Autodesk Inventor part; units mm, degrees
ref_plane "Work Plane2" through (12.9398, -24.5988, -20.5) normal (0, 0, 1) x (0.7071087, 0.7071049, 0)
ref_plane "YZ Plane" through (0, 0, 0) normal (1, 0, 0) x (0, 1, 0)
ref_plane "XZ Plane" through (0, 0, 0) normal (0, 1, 0) x (-1, 0, 0)
ref_plane "Work Plane1" through (69.3531, 0, -24) normal (0, 0, -1) x (-0.9792327, -0.2027397, 0)
sketch "Sketch1" plane through (69.3531, 0, -24) normal (0, 0, -1) x (-0.9792327, -0.2027397, 0)
  circle A0 centre (8.0687, 11.3576) radius 25.9979
  circle A1 centre (8.0703, 11.3562) radius 3.8103
  circle A2 centre (8.0703, 11.3562) radius 5
  point P0 (67.9128, 14.0606)
  dimension "d0" = 10
extrude "Extrusion1" add sketch "Sketch1" along normal blind 4 contours A0
sketch "Sketch2" plane through (59.1493, 9.4859, -28) normal (0, 0, -1) x (-1, 0, 0)
  line L0 (59.1493, -50.593) -> (59.1493, 54.0449)
  line L1 (-54.0467, -9.4859) -> (50.5907, -9.4859)
  line L2 (-15.9479, -15.1669) -> (4.4725, 20.2023)
  line L3 (4.4725, 20.2023) -> (19.4213, 5.2535)
  line L4 (19.4213, 5.2535) -> (-15.9479, -15.1669)
  line L5 (-39.0985, 39.0967) -> (35.6425, -35.6447)
  line L6 (-0.781, 0) -> (9.2905, 10.0715)
  line L7 (-0.781, 0) -> (13.4622, 0) construction
  line L8 (-15.9479, -15.1669) -> (-0.781, 0)
  circle A0 centre (4.4725, 20.2023) radius 1.6
  circle A1 centre (19.4213, 5.2535) radius 1.6
  circle A2 centre (-15.9479, -15.1669) radius 1.6 construction
  circle A3 centre (-16.8292, -16.048) radius 1.5
  dimension "d17" = 18
  dimension "d18" = 22
  dimension "d19" = 30
  dimension "d20" = 45
  dimension "d21" = 15
  dimension "d22" = 3.2
  dimension "d23" = 3.2
  dimension "d24" = 3.2
  dimension "d39" = 3
extrude "Extrusion2" cut sketch "Sketch2" against normal blind 3.4 contours A3 L8 L2 | L2 L4 A3 | A3 L4 L8 | A0 L3 L2 | L2 L3 A0 | A1 L3 L4 | L4 L3 A1
sketch "Sketch3" plane through (59.1493, 9.4859, -28) normal (0, 0, -1) x (-1, 0, 0)
  line L0 (-35.7047, 22.4019) -> (13.1872, -35.1292)
  line L1 (32.542, -18.6808) -> (-16.3499, 38.8503)
  line L2 (40.2702, -21.1784) -> (-21.1782, 40.2703)
  line L3 (-21.1782, 40.2703) -> (-40.2702, 21.1784)
  line L4 (-40.2702, 21.1784) -> (21.1782, -40.2703)
  line L5 (21.1782, -40.2703) -> (40.2702, -21.1784)
  line L6 (40.2702, -21.1784) -> (-40.2702, 21.1784) construction
  line L7 (-21.1782, 40.2703) -> (21.1782, -40.2703) construction
  point P0 (0, 0)
  dimension "d16" = 27
extrude "Extrusion3" cut sketch "Sketch3" against normal blind 1.5
sketch "Sketch4" plane through (69.3531, 0, -28) normal (0, 0, -1) x (-0.9792327, -0.2027397, 0)
  circle A0 centre (0.0169, -1.5448) radius 2
extrude "Extrusion4" cut sketch "Sketch4" against normal blind 25.4
sketch "Sketch6" plane through (69.3531, 0, -28) normal (0, 0, -1) x (-0.9792327, -0.2027397, 0)
  line L0 (-28.7292, -8.8539) -> (-25.804, -10.7757)
  line L1 (-20.2187, 4.1006) -> (-28.7292, -8.8539)
  line L2 (-20.2187, 4.1006) -> (-17.2935, 2.1789)
  circle A0 centre (-5.1575, -7.7691) radius 1.5
  line L3 (0.0784, 0.4542) -> (-17.9131, 12.2738)
  arc A1 (-17.9131, 12.2738) -> (19.2256, -12.1245) centre (8.0687, 11.3576) ccw
  line L4 (-28.7292, -8.8539) -> (-20.2187, 4.1006)
  line L5 (-20.2187, 4.1006) -> (-38.152, 15.8819)
  line L6 (-38.152, 15.8819) -> (-46.6625, 2.9274)
  line L7 (-46.6625, 2.9274) -> (-28.7292, -8.8539)
  line L8 (-52.6907, 6.8876) -> (-44.1802, 19.8422)
  line L9 (-44.1802, 19.8422) -> (-14.4793, 0.3302)
  line L10 (-37.9848, 15.7721) -> (-46.4954, 2.8175)
  line L11 (-46.4954, 2.8175) -> (-42228058.7703, 27741750.5128)
  line L12 (-42228058.7703, 27741750.5128) -> (-52.6907, 6.8876)
  line L13 (-14.4793, 0.3302) -> (-37.9848, 15.7721)
  circle A2 centre (-5.1575, -7.7691) radius 1.5
  circle A3 centre (-5.1575, -7.7691) radius 1.7
  circle A4 centre (26.0215, 20.4395) radius 2.75
  circle A5 centre (8.3525, 32.0472) radius 2.45
  circle A6 centre (26.0215, 20.4395) radius 1.6
  circle A7 centre (8.3525, 32.0472) radius 1.6
  arc A8 (0.0784, 0.4542) -> (1.8272, -0.6947) centre (0.0169, -1.5448) ccw
  line L14 (19.2256, -12.1245) -> (1.8272, -0.6947)
  point P0 (67.9128, 14.0606)
  point P1 (8.0213, -4.7639)
  point P2 (-4.9332, 3.7467)
  dimension "d44" = 0
  dimension "d47" = 0
  dimension "d48" = 3.4
  dimension "d49" = 3.2
  dimension "d50" = 3.2
extrude "Extrusion6" add sketch "Sketch6" along normal blind 4 contours A8 L14 A1 L3 | A3
sketch "Sketch7" plane through (69.3531, 0, -32) normal (0, 0, -1) x (-0.9792327, -0.2027397, 0)
  circle A0 centre (-5.1575, -7.7691) radius 2.45
  circle A1 centre (8.3525, 32.0472) radius 2.75
  circle A2 centre (26.0215, 20.4395) radius 2.75
  point P0 (67.9128, 14.0606)
hole "Hole1" at (39.7281, 14.7395, -32) at (54.6768, 29.6883, -32) at (75.9786, -6.5621, -32) direction (0, 0, 1) diameter 3.4 end through all counterbore diameter 5 counterbore depth 3
sketch "Sketch8" plane through (69.3531, 0, -32) normal (0, 0, -1) x (-0.9792327, -0.2027397, 0)
  line L0 (22.3699, -1.0133) -> (13.834, 4.5943)
  line L1 (13.834, 4.5943) -> (22.3444, 17.5489)
  line L2 (30.8803, 11.9413) -> (22.3444, 17.5489)
  line L3 (22.3699, -1.0133) -> (30.8803, 11.9413)
  line L4 (29.1977, -5.4988) -> (37.7081, 7.4558)
  line L5 (29.1977, -5.4988) -> (22.3699, -1.0133)
  line L6 (37.7081, 7.4558) -> (30.8803, 11.9413)
  line L7 (29.1977, -5.4988) -> (37.7081, 7.4558)
  line L8 (37.7081, 7.4558) -> (48.711, 0.2276)
  line L9 (48.711, 0.2276) -> (40.2006, -12.7271)
  line L10 (40.2006, -12.7271) -> (29.1977, -5.4988)
  point P0 (67.9128, 14.0606)
  point P1 (11.3572, 0.3138)
  point P2 (-1.5974, 8.8243)
  point P3 (14.9357, 6.2713)
ref_plane "Work Plane2" through (12.9398, -24.5988, -20.5) normal (0, 0, 1) x (0.7071087, 0.7071049, 0)
extrude "Extrusion7" cut sketch "Sketch8" against normal up to surface (11.5 mm away) contours L3 L6 L4 L5
properties part number "Matchboxscope_sample_v0"
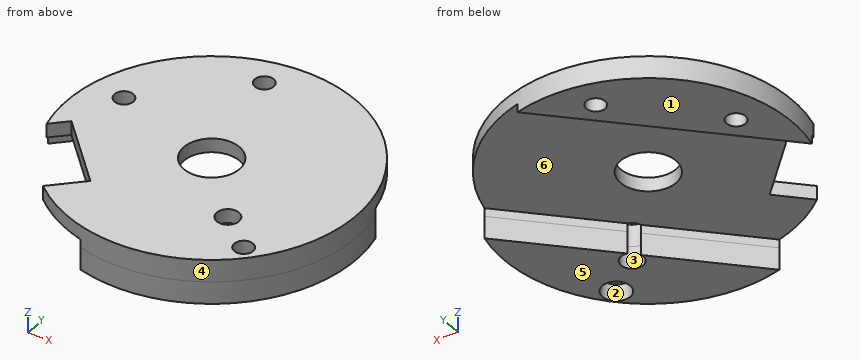
Can you work these out from the model? Positions are in its coordinate system, mm. Face numbers are marked on the shaded views. A direction names the side the tool comes from. Give positions to 0.01 mm unless a question says otherwise; leave off trailing zeros. Order: outer loops, then holes, each group sorted by start corner. A loop starts at its lowest first (then second) coordinate and runs counter-clockwise, first axis right, second up. Notation, with made-up numbers: M 5.25,-14 L 16.25,-14 A22 ccw 16.25,-2 Z; hole C 39,-19 d11. An arc over 180 degrees is marked long. Use one line per item in the form item = value.
Item 1: If we section it at A-A, the plane x = 68.5: Write out the boundary of the cut face in (y, z), and give its area (3 significant figures).
Values follow:
outline = M -14.77,-32 L -3.15,-32 L -3.15,-24 L -14.77,-24 Z; M 0.12,-26.5 L 33.74,-26.5 L 33.74,-24 L 0.12,-24 Z
area = 177 mm^2
Item 2: Will these pins go through, and if not, where does the flat tip stop? pin 1 Ø2 at (x, y) = (39.73, 14.74) entering from -Z; pin 2 Ø8 at (x, y) = (40, 9.5) entering from -Z; pin 3 Ø4 at (x, z) = (79.5, -30.5) entering from +Y; pin 4 Ø1 at (y, z) = (23, -26.5) entering from -X.
Values follow:
pin_1 = through
pin_2 = -28
pin_3 = 12.74
pin_4 = 36.64
Item 3: If we section it at B-B, the plane z = -31: Write out the boundary of the cut face in (x, y), and give its area (3 significant figures).
Values follow:
outline = M 52.98,-15.77 A26 ccw 84.41,15.65 L 69.18,0.43 A2 cw long 67.7,-1.05 Z; hole C 75.98,-6.56 d5
area = 361 mm^2
Item 4: For the marked faces 1, 2 and 3, which set-ups out of +Z, -Z, +X, -X, +Y, -Y let a thin tool reach every point of the face, with its end or its side?
Values follow:
face_1 = -Z, -X, +Y
face_2 = -Z
face_3 = +Z, -Z
Item 5: If I drill on line 1 along Z through (x, y) = (44, 22); line 2 along Y through (x, z) = (60, -26.25); line 3 along Z through (x, y) = (60, -4), over which ranges is the centre line in solid material (lowest first)? Write a range as [from, to].
Values follow:
line_1 = [-28, -24]
line_2 = [-16.5, 4.56], [14.41, 35.47]
line_3 = [-26.5, -24]
Item 6: Thinking about a two-plate mould opening in Y: for the marked faces 4, 5 and 6, which applies, pulls with the +Y half, pulls with the -Y half, needs draft (parallel to the pull), parting line crosses it, or undercut?
Values follow:
face_4 = parting line crosses it
face_5 = needs draft
face_6 = undercut
Item 7: If we section it at C-C, the plane y = 6.5: Write out the boundary of the cut face in (x, z), and give its area (3 significant figures).
Values follow:
outline = M 33.32,-28 L 37.07,-28 L 37.07,-26.5 L 55.14,-26.5 L 55.14,-24 L 33.32,-24 Z; M 63.16,-26.5 L 75.26,-26.5 L 75.26,-32 L 84.98,-32 L 84.98,-24 L 63.16,-24 Z
area = 168 mm^2
